from build123d import *

# Parameters (mm, degrees)
F1_DEPTH = 600
F3_DEPTH = 150
F5_DEPTH = 600.001
F6_R     = 200
F7_DEPTH = 550.001


with BuildPart() as f1:
    # F0 (on Front) → F1 (new body)
    with BuildSketch(Plane.XZ):
        Polygon((302.476975, 1044.568934), (302.476975, 794.568934), (1502.476975, 794.568934), (1502.476975, 1044.568934), (1202.476975, 1044.568934), (1202.476975, 1344.568934), (602.476975, 1344.568934), (602.476975, 1044.568934), align=None)
    extrude(amount=F1_DEPTH)

    # F2 (on face) → F3 (join)
    with BuildSketch(Plane(origin=(0, 0, 0), x_dir=(-1, 0, 0), z_dir=(0, 1, 0))):
        Polygon((-1202.476975, 1344.568934), (-1502.476975, 1044.568934), (-1202.476975, 1044.568934), align=None)
        Polygon((-302.476975, 1044.568934), (-602.476975, 1344.568934), (-602.476975, 1044.568934), align=None)
    extrude(amount=-F3_DEPTH)

    # F4 (on face) → F5 (cut, through all)
    with BuildSketch(Plane.XZ.offset(600)):
        with BuildLine():
            Line((952.476975, 445.364194), (952.476975, 1057.966394))
            ThreePointArc((952.476975, 1057.966394), (902.476975, 1244.568934), (852.476975, 1057.966394))
            Line((852.476975, 1057.966394), (852.476975, 445.364194))
            Line((852.476975, 445.364194), (952.476975, 445.364194))
        make_face()
    extrude(amount=-F5_DEPTH, mode=Mode.SUBTRACT)

    # F6 (on face) → F7 (cut, through all)
    with BuildSketch(Plane.XY.offset(1344.568934)):
        with Locations((902.476975, -300)):
            Circle(F6_R)
    extrude(amount=-F7_DEPTH, mode=Mode.SUBTRACT)


solid = f1.part
Could you check a few things on this model? Use its own coordinates, in mm. A direction names the side the tool comes from. Coordinates: 2 decimals unless noted, no trailing zeros. Loops run counter-clockwise (first coordinate to the right, second up) from the corner with the lowest first, then second, coordinate; pieces in that order, holes last.
1. Imagine slicing it at A-A (z = 835). Please give me the cut outline in (x, y), and give its area (3 significant figures).
2. Imagine slicing it at C-C (x = 891). Please give me the cut outline in (y, z).
3. Imagine slicing it at B-B (y = -372.5). Please give me the cut outline in (x, z), and give its area (3 significant figures).
4. I need wall thicknesses on L1, parallel to X at y = -509, z = 977.5; L2, parallel to Z at x = 1231, y = -264; L3, parallel to Y at x = 1269, z = 1220. Which ranges of each line are inside material? Lowest first, please.
5. For faces 5 (the face through (1355, -372, 1044.569)), 6 (the face through (521, -150, 1130)), 7 (the face through (1285, -296, 794.569)), 8 (the face through (852.477, -54, 928)), 9 (the face through (1093.241, -239.925, 1073.419)), which set-ups out of +Z, -Z, +X, -X, +Y, -Y let a thin tool reach every point of the face, with its end or its side?
6. For P1, Ø1.5, axis at x = 863.5, y = -494.5, coming from the +Z side; P2, Ø8, axis at y = -85.5, z = 1221, coming from the +X side; P3, Ø2, axis at y = -360, z = 1138.5, coming from the +X side, each with a flat end and sliding along its axis, tell me the tip position at first contact or that it passes through.
7. Imagine slicing it at D-D (x = 398.5). Please give me the cut outline in (y, z), and give its area (3 significant figures).
8. We'd pull the mould along X, two halves only. Please class faces 1 (the face through (1502.477, -296, 918)), 2 (the face through (952.477, -54, 924)), 3 (the face through (602.477, -372, 1197)), 4 (the face through (778, 0, 1073)): released by +X, released by -X, zero draft, split by the parting line, or undercut.
Computed values:
1. outline: (302.48, -600) - (852.48, -600) - (852.48, -493.65) arc R200 cw to (852.48, -106.35) - (852.48, 0) - (302.48, 0) - close; (952.48, -600) - (1502.48, -600) - (1502.48, 0) - (952.48, 0) - (952.48, -106.35) arc R200 cw to (952.48, -493.65) - close
1. area: 574,000 mm2
2. outline: (-600, 1243.91) - (-499.67, 1243.91) - (-499.67, 1344.57) - (-600, 1344.57) - close; (-100.33, 1243.91) - (0, 1243.91) - (0, 1344.57) - (-100.33, 1344.57) - close
3. outline: (302.48, 794.57) - (716.08, 794.57) - (716.08, 1344.57) - (602.48, 1344.57) - (602.48, 1044.57) - (302.48, 1044.57) - close; (1088.87, 794.57) - (1502.48, 794.57) - (1502.48, 1044.57) - (1202.48, 1044.57) - (1202.48, 1344.57) - (1088.87, 1344.57) - close
3. area: 275,000 mm2
4. L1: x = 302.48 to 852.48, 952.48 to 1502.48
4. L2: z = 794.57 to 1044.57
4. L3: y = -150 to 0
5. face 5: +Z, +X, -Y
5. face 6: +Z, -X, -Y
5. face 7: -Z, +X, -X, +Y, -Y
5. face 8: -Z, +Y, -Y
5. face 9: +Z, -Z
6. P1: passes through
6. P2: stops at x = 1330.05
6. P3: stops at x = 1202.48
7. outline: (-600, 794.57) - (0, 794.57) - (0, 1140.59) - (-150, 1140.59) - (-150, 1044.57) - (-600, 1044.57) - close
7. area: 164,000 mm2
8. face 1: released by +X
8. face 2: undercut
8. face 3: released by -X
8. face 4: zero draft
